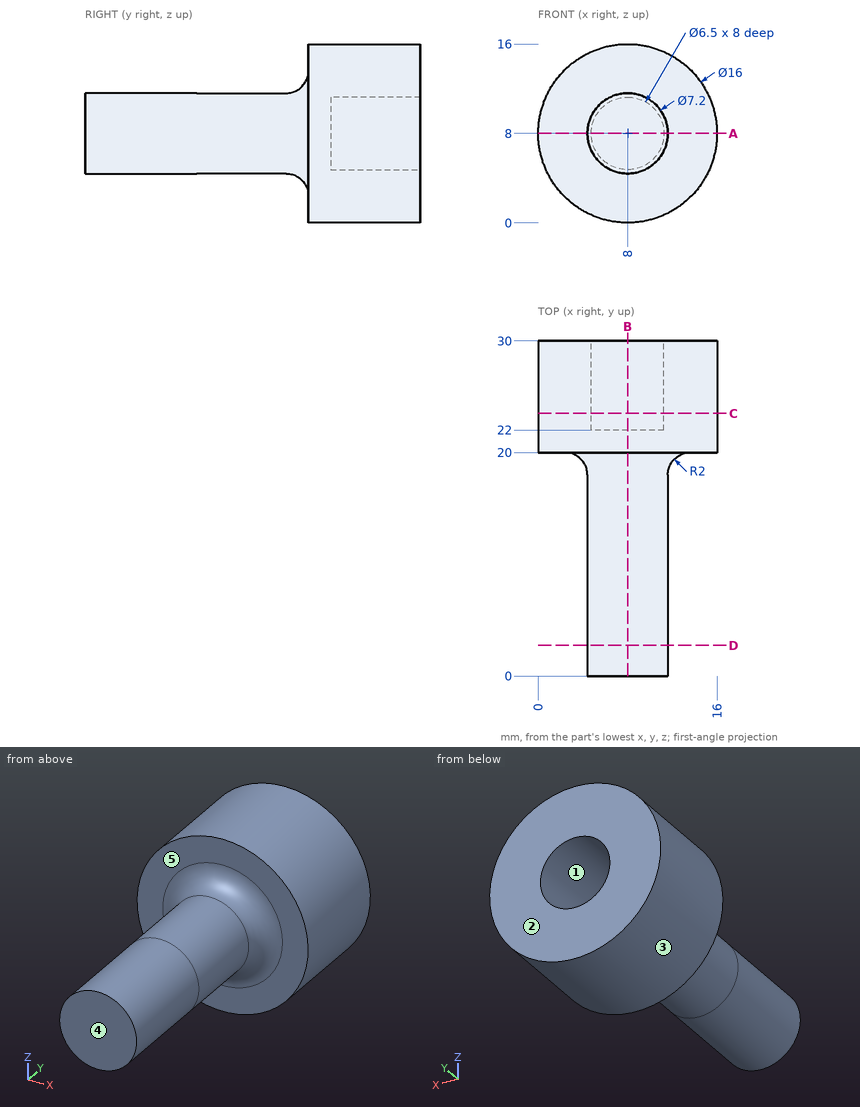
For this review, use the dimensioned drawing (mm, ordinates from the lowest corner) and the shaded views. A direction names the side the tool comes from. Coordinates: 2 decimals unless noted, no trailing zeros. Loops run counter-clockwise (first coordinate to the right, second up) from the corner with the lowest first, then second, coordinate; pieces in that order, holes last.
1. For the marked faces 4 and 5, list the 3-axis set-ups (+Z, -Z, +X, -X, +Y, -Y) from which the entire face can be reached by the end or side of a thin tool; tool diameter is ignored.
2. Mouldability with a two-part tool opening along Z and no side actions: class the marked faces 1, 2 and 3 as +Z half, -Z half, draft (parallel to the pull), parting line (faces both ways), or undercut.
3. Insertion check: P1, Ø5, axis at y = 8.5, z = 8, coming from the +X side; P2, Ø1.5, axis at y = 6, z = 2.5, coming from the +X side; P3, Ø8, axis at x = 11.5, y = 6, coming from the -Z side. Each pin has a flat end and moves straight along its axis. Give the tip position at first contact, or say it passes through.
4. Add section C-C, the plane y = 23.5. Give the boundary of the cut face in (x, z), then the cut area to 3 significant figures.
5. Add section B-B, the plane x = 8. Give the boundary of the cut face in (y, z), then the cut area to 3 significant figures.
6. For line 1 (X direction, y = 26.5, z = 8); line 2 (Y direction, x = 3, z = 5.25); line 3 (Y direction, x = 10.5, z = 8.5), list the stretches that pass through material, from the lowest coordinate up.
7. Add section D-D, the plane y = 2.75. Give the boundary of the cut face in (x, z).
8. Add section A-A, the plane z = 8. Give the boundary of the cut face in (x, y).
Result:
1. face 4: +Z, -Z, +X, -X, -Y
1. face 5: -Y
2. face 1: undercut
2. face 2: draft
2. face 3: parting line
3. P1: stops at x = 11.6
3. P2: passes through
3. P3: stops at z = 4.4
4. outline: circle Ø16 at (8, 8); hole circle Ø6.5 at (8, 8)
4. area: 168 mm2
5. outline: (0, 4.4) - (18, 4.4) arc R2 cw to (20, 2.4) - (20, 0) - (30, 0) - (30, 4.75) - (22, 4.75) - (22, 11.25) - (30, 11.25) - (30, 16) - (20, 16) - (20, 13.6) arc R2 cw to (18, 11.6) - (0, 11.6) - close
5. area: 254 mm2
6. line 1: x = 0 to 4.75, 11.25 to 16
6. line 2: y = 20 to 30
6. line 3: y = 0 to 22
7. outline: circle Ø7.2 at (8, 8)
8. outline: (0, 20) - (2.4, 20) arc R2 cw to (4.4, 18) - (4.4, 0) - (11.6, 0) - (11.6, 18) arc R2 cw to (13.6, 20) - (16, 20) - (16, 30) - (11.25, 30) - (11.25, 22) - (4.75, 22) - (4.75, 30) - (0, 30) - close
